Geometry check sheet. Reference: the model listing, model coordinates, mm. Give positions to 0.01 mm unless a question says otherwise; leave off trailing zeros. Order: outer loops, then holes, each group sorted by start corner. A loop starts at its lowest first (then second) coordinate and runs counter-clockwise, first axis right, second up.
from build123d import *

# Parameters (mm, degrees)
ESQUISSE1_W             = 60
ESQUISSE1_H             = 60
BOSS_EXTRU_1_DEPTH      = 2
ESQUISSE4_R             = 3
ESQUISSE4_R_2           = 2
ENL_V_MAT_EXTRU_1_DEPTH = 10
ESQUISSE5_R             = 2
ENL_V_MAT_EXTRU_2_DEPTH = 10
ESQUISSE12_R            = 2
ENL_V_MAT_EXTRU_5_DEPTH = 2


with BuildPart() as part:
    # Esquisse1 → Boss.-Extru.1 (new body)
    with BuildSketch(Plane(origin=(0, 0, 0), x_dir=(1, 0, 0), z_dir=(0, 1, 0))):
        with Locations((30, 30)):
            Rectangle(ESQUISSE1_W, ESQUISSE1_H)
    extrude(amount=BOSS_EXTRU_1_DEPTH)

    # Esquisse4 → Enlèv. mat.-Extru.1 (cut)
    with BuildSketch(Plane(origin=(0, 2, 0), x_dir=(1, 0, 0), z_dir=(0, 1, 0))):
        with Locations(Location((10.5, 20, 0), (0, 0, 270))):  # turned: the seam where the file's is
            Circle(ESQUISSE4_R)
        with Locations(Location((20.5, 20, 0), (0, 0, 270))):  # turned: the seam where the file's is
            Circle(ESQUISSE4_R)
        with Locations(Location((15.5, 10, 0), (0, 0, 270))):  # turned: the seam where the file's is
            Circle(ESQUISSE4_R_2)
    extrude(amount=-ENL_V_MAT_EXTRU_1_DEPTH, mode=Mode.SUBTRACT)

    # Esquisse5 → Enlèv. mat.-Extru.2 (cut)
    with BuildSketch(Plane(origin=(0, 2, 0), x_dir=(1, 0, 0), z_dir=(0, 1, 0))):
        with Locations(Location((5, 5, 0), (0, 0, 270))):  # turned: the seam where the file's is
            Circle(ESQUISSE5_R)
        with Locations(Location((55, 5, 0), (0, 0, 270))):  # turned: the seam where the file's is
            Circle(ESQUISSE5_R)
        with Locations(Location((55, 55, 0), (0, 0, 270))):  # turned: the seam where the file's is
            Circle(ESQUISSE5_R)
        with Locations(Location((5, 55, 0), (0, 0, 270))):  # turned: the seam where the file's is
            Circle(ESQUISSE5_R)
        with Locations(Location((30, 55, 0), (0, 0, 270))):  # turned: the seam where the file's is
            Circle(ESQUISSE5_R)
        with Locations(Location((30, 5, 0), (0, 0, 270))):  # turned: the seam where the file's is
            Circle(ESQUISSE5_R)
        with Locations(Location((30, 30, 0), (0, 0, 270))):  # turned: the seam where the file's is
            Circle(ESQUISSE5_R)
        with Locations(Location((55, 30, 0), (0, 0, 270))):  # turned: the seam where the file's is
            Circle(ESQUISSE5_R)
        with Locations(Location((5, 30, 0), (0, 0, 270))):  # turned: the seam where the file's is
            Circle(ESQUISSE5_R)
    extrude(amount=-ENL_V_MAT_EXTRU_2_DEPTH, mode=Mode.SUBTRACT)

    # Esquisse12 → Enlèv. mat.-Extru.5 (cut)
    with BuildSketch(Plane(origin=(0, 2, 0), x_dir=(1, 0, 0), z_dir=(0, 1, 0))):
        with Locations(Location((17.5, 55, 0), (0, 0, 270))):  # turned: the seam where the file's is
            Circle(ESQUISSE12_R)
        with Locations(Location((42.5, 55, 0), (0, 0, 270))):  # turned: the seam where the file's is
            Circle(ESQUISSE12_R)
        with Locations(Location((42.5, 42.5, 0), (0, 0, 270))):  # turned: the seam where the file's is
            Circle(ESQUISSE12_R)
        with Locations(Location((17.5, 42.5, 0), (0, 0, 270))):  # turned: the seam where the file's is
            Circle(ESQUISSE12_R)
        with Locations(Location((42.5, 17.5, 0), (0, 0, 270))):  # turned: the seam where the file's is
            Circle(ESQUISSE12_R)
        with Locations(Location((55, 17.5, 0), (0, 0, 270))):  # turned: the seam where the file's is
            Circle(ESQUISSE12_R)
        with Locations(Location((55, 42.5, 0), (0, 0, 270))):  # turned: the seam where the file's is
            Circle(ESQUISSE12_R)
        with Locations(Location((42.5, 5, 0), (0, 0, 270))):  # turned: the seam where the file's is
            Circle(ESQUISSE12_R)
        with Locations(Location((42.5, 30, 0), (0, 0, 270))):  # turned: the seam where the file's is
            Circle(ESQUISSE12_R)
        with Locations(Location((5, 42.5, 0), (0, 0, 270))):  # turned: the seam where the file's is
            Circle(ESQUISSE12_R)
        with Locations(Location((30, 42.5, 0), (0, 0, 270))):  # turned: the seam where the file's is
            Circle(ESQUISSE12_R)
        with Locations(Location((30, 17.5, 0), (0, 0, 270))):  # turned: the seam where the file's is
            Circle(ESQUISSE12_R)
    extrude(amount=-ENL_V_MAT_EXTRU_5_DEPTH, mode=Mode.SUBTRACT)


solid = part.part
Item 1: Sectioned sample at B-B (x = 20.5). Enter the section's corners in (y, z), and give its area (3 significant figures).
Reported:
outline: (0, -60) - (2, -60) - (2, -23) - (0, -23) - close; (0, -17) - (2, -17) - (2, 0) - (0, 0) - close
area: 108 mm2
Item 2: Sectioned sample at A-A (z = -30). Enter the section's corners in (x, y).
Reported:
outline: (0, 0) - (3, 0) - (3, 2) - (0, 2) - close; (7, 0) - (28, 0) - (28, 2) - (7, 2) - close; (32, 0) - (40.5, 0) - (40.5, 2) - (32, 2) - close; (44.5, 0) - (53, 0) - (53, 2) - (44.5, 2) - close; (57, 0) - (60, 0) - (60, 2) - (57, 2) - close
Item 3: Sectioned sample at C-C (z = -42.5). Enter the section's corners in (x, y), and give its area (3 significant figures).
Reported:
outline: (0, 0) - (3, 0) - (3, 2) - (0, 2) - close; (7, 0) - (15.5, 0) - (15.5, 2) - (7, 2) - close; (19.5, 0) - (28, 0) - (28, 2) - (19.5, 2) - close; (32, 0) - (40.5, 0) - (40.5, 2) - (32, 2) - close; (44.5, 0) - (53, 0) - (53, 2) - (44.5, 2) - close; (57, 0) - (60, 0) - (60, 2) - (57, 2) - close
area: 80.0 mm2
Item 4: Sectioned sample at D-D (y = 1.7). Give the number of separate pieces and of enclosed holes in the cut face, and give its area (3 significant figures).
Reported:
separate pieces: 1
enclosed holes: 24
area: 3,270 mm2
Item 5: Draft check along Z on faces 1 (the cylindrical face through (28.226, 1.014, -29.077)), 2 (the flat face through (30, 1, -60)), 3 (the flat face through (60, 1, -30)). Enter one of: released by +Z, released by -Z, zero draft, split by the parting line, or undercut.
Reported:
face 1: undercut
face 2: released by -Z
face 3: zero draft
Item 6: Scan lines: L1, parallel to X at y = 0.95, z = -30; L2, parallel to X at y = 1, z = -55; L3, parallel to X at y = 0.8, z = -18. Record each from-to range of solid material in increasing order.
Reported:
L1: x = 0 to 3, 7 to 28, 32 to 40.5, 44.5 to 53, 57 to 60
L2: x = 0 to 3, 7 to 15.5, 19.5 to 28, 32 to 40.5, 44.5 to 53, 57 to 60
L3: x = 0 to 8.26, 12.74 to 18.26, 22.74 to 28.06, 31.94 to 40.56, 44.44 to 53.06, 56.94 to 60
